Autodesk Inventor part; units mm, degrees
ref_plane "YZ Plane" through (0, 0, 0) normal (1, 0, 0) x (0, 1, 0)
ref_plane "XZ Plane" through (0, 0, 0) normal (0, 1, 0) x (-1, 0, 0)
ref_plane "XY Plane" through (0, 0, 0) normal (0, 0, 1) x (1, 0, 0)
sketch "Sketch1" plane through (0, 0, 0) normal (0, 0, 1) x (1, 0, 0)
  circle A0 centre (0, 0) radius 17.5
  circle A1 centre (0, 0) radius 67.5
  circle A2 centre (41.5, 0) radius 2
  circle A3 centre (29.3449, 29.3449) radius 2
  circle A4 centre (0, 41.5) radius 2
  circle A5 centre (-29.3449, 29.3449) radius 2
  circle A6 centre (-41.5, 0) radius 2
  circle A7 centre (-29.3449, -29.3449) radius 2
  circle A8 centre (0, -41.5) radius 2
  circle A9 centre (29.3449, -29.3449) radius 2
  dimension "d0" = 35
  dimension "d1" = 135
  dimension "d2" = 4
  dimension "d3" = 41.5
  dimension "d6" = 360
extrude "Extrusion1" add sketch "Sketch1" along normal blind 15
sketch "Sketch5" plane through (0, 0, 15) normal (0, 0, 1) x (1, 0, 0)
  circle A0 centre (0, 0) radius 67.5
  circle A1 centre (0, 0) radius 48.5
  dimension "d19" = 97
extrude "Extrusion4" add sketch "Sketch5" along normal blind 40
sketch "Sketch11" plane through (0, 0, 55) normal (0, 0, 1) x (1, 0, 0)
  line L0 (0, 77.9423) -> (67.5, 38.9711)
  line L1 (67.5, 38.9711) -> (67.5, -38.9711)
  line L2 (67.5, -38.9711) -> (0, -77.9423)
  line L3 (0, -77.9423) -> (-67.5, -38.9711)
  line L4 (-67.5, -38.9711) -> (-67.5, 38.9711)
  line L5 (-67.5, 38.9711) -> (0, 77.9423)
  circle A0 centre (0, 0) radius 67.5
extrude "Extrusion8" add sketch "Sketch11" against normal blind 55 contours L0 A0 L5 | L0 L1 A0 | A0 L4 L5 | L1 L2 A0 | A0 L3 L4 | L2 L3 A0
sketch "Sketch16" plane through (0, 0, 15) normal (0, 0, 1) x (1, 0, 0)
  circle A0 centre (-41.5, 0) radius 2
  circle A1 centre (0, 0) radius 34.5
  circle A2 centre (0, 0) radius 48.5
  line L0 (-48.5, 0) -> (-34.5, 0)
  circle A3 centre (0, 0) radius 48.5
extrude "Extrusion11" cut sketch "Sketch16" against normal blind 8
sketch "Sketch19" plane through (0, 0, 55) normal (0, 0, 1) x (1, 0, 0)
  circle A0 centre (0, 0) radius 48.5
  line L0 (0, -77.9423) -> (-67.5, -38.9711)
  line L1 (67.5, -38.9711) -> (0, -77.9423)
  line L2 (67.5, 38.9711) -> (67.5, -38.9711)
  line L3 (0, 77.9423) -> (67.5, 38.9711)
  line L4 (-67.5, 38.9711) -> (0, 77.9423)
  line L5 (-67.5, -38.9711) -> (-67.5, 38.9711)
  line L6 (0, 68.1273) -> (59, 34.0637)
  line L7 (59, 34.0637) -> (59, -34.0637)
  line L8 (59, -34.0637) -> (0, -68.1273)
  line L9 (0, -68.1273) -> (-59, -34.0637)
  line L10 (-59, -34.0637) -> (-59, 34.0637)
  line L11 (-59, 34.0637) -> (0, 68.1273)
  dimension "d58" = 118
extrude "Extrusion13" cut sketch "Sketch19" against normal through all contours L0 L5 L4 L3 L2 L1
sketch "Sketch20" plane through (0, 0, 0) normal (0, 0, -1) x (-1, 0, 0)
  line L0 (-59, -34.0637) -> (-59, -115)
  line L1 (-59, -115) -> (59, -115)
  line L2 (59, -34.0637) -> (59, 34.0637)
  line L3 (59, -115) -> (59, -34.0637)
  line L4 (-59, -34.0637) -> (0, -68.1273)
  line L5 (0, -68.1273) -> (59, -34.0637)
  line L6 (-59, -34.0637) -> (0, -68.1273)
  line L7 (0, -68.1273) -> (59, -34.0637)
  point P0 (0, 0)
  dimension "d61" = 115
extrude "Extrusion14" add sketch "Sketch20" against normal blind 55
sketch "Sketch22" plane through (0, 0, 55) normal (0, 0, 1) x (1, 0, 0)
  line L0 (59, -115) -> (59, 34.0637) construction
  line L1 (59, 34.0637) -> (0, 68.1273) construction
  line L2 (0, 68.1273) -> (-59, 34.0637) construction
  line L3 (-59, 34.0637) -> (-59, -115) construction
  line L4 (-59, -115) -> (59, -115) construction
  line L5 (52, 30.0222) -> (52, -108) construction
  line L6 (52, -108) -> (-52, -108) construction
  line L7 (-52, -108) -> (-52, 30.0222) construction
  line L8 (-52, 30.0222) -> (0, 60.0444) construction
  line L9 (0, 60.0444) -> (52, 30.0222) construction
  circle A0 centre (-52, -108) radius 2
  circle A1 centre (52, -108) radius 2
  circle A2 centre (0, 60.0444) radius 2
  circle A3 centre (-52, 30.0222) radius 2
  circle A4 centre (52, 30.0222) radius 2
  circle A5 centre (-26, -108) radius 2
  circle A6 centre (26, -108) radius 2
  circle A7 centre (0, -108) radius 2
  circle A8 centre (-52, -68.9889) radius 2
  circle A9 centre (-52, -38.9889) radius 2
  circle A10 centre (-52, 0) radius 2
  circle A11 centre (52, 0) radius 2
  circle A12 centre (52, -38.9889) radius 2
  circle A13 centre (52, -68.9889) radius 2
  circle A14 centre (-26, 45.0333) radius 2
  circle A15 centre (26, 45.0333) radius 2
  point P0 (0, 0)
  point P1 (0, 0)
  point P2 (0, 68.1273)
  point P3 (59, 34.0637)
  dimension "d64" = 7
  dimension "d65" = 4
  dimension "d66" = 4
  dimension "d67" = 4
  dimension "d68" = 4
  dimension "d69" = 4
  dimension "d70" = 4
  dimension "d71" = 4
  dimension "d72" = 4
  dimension "d73" = 4
  dimension "d74" = 4
  dimension "d75" = 4
  dimension "d76" = 4
  dimension "d77" = 4
  dimension "d78" = 4
  dimension "d79" = 4
  dimension "d80" = 4
  dimension "d81" = 30
extrude "Extrusion15" cut sketch "Sketch22" against normal through all contours A0 | A1 | A3 | A4 | A9 | A12 | A14 | A15
sketch "Sketch23" plane through (-59, -115, 0) normal (0, -1, 0) x (1, 0, 0)
  line L0 (12.812, 40) -> (35.906, 80)
  line L1 (35.906, 80) -> (82.094, 80)
  line L2 (82.094, 80) -> (105.188, 40)
  line L3 (105.188, 40) -> (82.094, 0)
  line L4 (82.094, 0) -> (35.906, 0)
  line L5 (35.906, 0) -> (12.812, 40)
  line L6 (118, 0) -> (0, 0)
  point P0 (59, 0)
  point P1 (59, 40)
  point P2 (59, 0)
  point P3 (59, 0)
  dimension "d87" = 80
extrude "Extrusion16" add sketch "Sketch23" along normal blind 13
sketch "Sketch24" plane through (-59, -128, 0) normal (0, -1, 0) x (1, 0, 0)
  line L0 (35.906, 80) -> (12.812, 40)
  line L1 (12.812, 40) -> (35.906, 0)
  line L2 (35.906, 0) -> (82.094, 0)
  line L3 (82.094, 0) -> (105.188, 40)
  line L4 (105.188, 40) -> (82.094, 80)
  line L5 (82.094, 80) -> (35.906, 80)
  line L6 (40.5248, 8) -> (22.0496, 40)
  line L7 (22.0496, 40) -> (40.5248, 72)
  line L8 (40.5248, 72) -> (77.4752, 72)
  line L9 (77.4752, 72) -> (95.9504, 40)
  line L10 (95.9504, 40) -> (77.4752, 8)
  line L11 (77.4752, 8) -> (40.5248, 8)
  point P0 (59, 0)
  dimension "d88" = 8
extrude "Extrusion17" cut sketch "Sketch24" against normal up to surface (13 mm away) from surface at 0
sketch "Sketch25" plane through (-59, -128, 0) normal (0, -1, 0) x (1, 0, 0)
  line L0 (95.9504, 40) -> (77.4752, 72)
  line L1 (77.4752, 72) -> (40.5248, 72)
  line L2 (40.5248, 72) -> (22.0496, 40)
  line L3 (22.0496, 40) -> (40.5248, 8)
  line L4 (40.5248, 8) -> (77.4752, 8)
  line L5 (77.4752, 8) -> (95.9504, 40)
  circle A0 centre (59, 40) radius 12
  point P0 (59, 0)
  point P1 (59, 72)
  dimension "d91" = 24
extrude "Extrusion18" cut sketch "Sketch25" against normal blind 40 contours A0
sketch "Sketch26" plane through (0, 0, 55) normal (0, 0, 1) x (1, 0, 0)
  line L0 (12, -88) -> (-12, -88)
  line L1 (12, -128) -> (-12, -128)
  line L2 (12, -88) -> (-12, -88)
  line L3 (-12, -88) -> (12, -88)
  line L4 (12, -88) -> (12, -101)
  line L5 (12, -101) -> (-12, -101)
  line L6 (-12, -101) -> (-12, -88)
  point P0 (0, 0)
  dimension "d94" = 13
extrude "Extrusion19" cut sketch "Sketch26" against normal blind 15
sketch "Sketch27" plane through (-36.9504, -128, 40) normal (-0.866, 0, 0.5) x (0.5, 0, 0.866)
  line L0 (17.3205, 13) -> (36.9504, 13)
  line L1 (17.3205, 13) -> (0, 13)
  line L2 (0, 0) -> (0, 13)
  line L3 (36.9504, 0) -> (0, 0)
  line L4 (36.9504, 0) -> (36.9504, 13)
  circle A0 centre (11.4041, 4) radius 2
  circle A1 centre (25.5463, 9) radius 2
  line L5 (11.4041, 4) -> (25.5463, 9) construction
  line L6 (0, 13) -> (36.9504, 13)
  point P0 (-16.1658, 128)
  point P1 (18.4752, 6.5)
  point P2 (18.4752, 13)
  point P3 (0, 6.5)
  dimension "d97" = 4
  dimension "d98" = 4
  dimension "d99" = 15
  dimension "d112" = 5
extrude "Extrusion20" cut sketch "Sketch27" against normal blind 20 contours A0 | A1
pattern_circular "Circular Pattern1" count 6 over 360 about axis through (0, -128, 40) along (0, 1, 0) of "Extrusion20"
sketch "Sketch28" plane through (0, 0, 55) normal (0, 0, 1) x (1, 0, 0)
  circle A0 centre (0, 53.1273) radius 2
  circle A1 centre (-34, -90) radius 2
  line L0 (-59, 34.0637) -> (-59, -115)
  line L1 (-59, -115) -> (-28.2902, -115)
  point P0 (0, 0)
  point P1 (0, 68.1273)
  dimension "d105" = 4
  dimension "d106" = 15
  dimension "d107" = 4
  dimension "d108" = 25
  dimension "d109" = 25
extrude "Extrusion21" cut sketch "Sketch28" against normal through all
sketch "Sketch30" plane through (0, 0, 55) normal (0, 0, 1) x (1, 0, 0)
  circle A0 centre (0, 0) radius 48.5 construction
  line L0 (12, -88) -> (12, -101) construction
  line L1 (12, -88) -> (-12, -88) construction
  line L2 (-12, -88) -> (-12, -101) construction
  line L3 (-12, -101) -> (12, -101) construction
  line L4 (12, -128) -> (-12, -128) construction
  circle A1 centre (-34, -90) radius 2 construction
  line L5 (-17, -83) -> (17, -83) construction
  line L6 (17, -83) -> (17, -106) construction
  line L7 (17, -106) -> (-17, -106) construction
  line L8 (-17, -106) -> (-17, -83) construction
  circle A2 centre (-34, -90) radius 7 construction
  circle A3 centre (0, 0) radius 53.5 construction
  circle A4 centre (0, 53.1273) radius 2 construction
  circle A5 centre (-34, -90) radius 2 construction
  line L9 (-12, -101) -> (-12, -88) construction
  line L10 (-12, -88) -> (12, -88) construction
  line L11 (12, -88) -> (12, -101) construction
  line L12 (12, -101) -> (-12, -101) construction
  circle A6 centre (26, 45.0333) radius 2 construction
  circle A7 centre (-52, 30.0222) radius 2 construction
  circle A8 centre (-52, -108) radius 2 construction
  circle A9 centre (52, -38.9889) radius 2 construction
  circle A10 centre (52, -108) radius 2 construction
  circle A11 centre (-52, -38.9889) radius 2 construction
  circle A12 centre (-26, 45.0333) radius 2 construction
  circle A13 centre (52, 30.0222) radius 2 construction
  line L13 (0, 68.1273) -> (-59, 34.0637) construction
  line L14 (-59, 34.0637) -> (-59, -115) construction
  line L15 (-59, -115) -> (-28.2902, -115) construction
  line L16 (-28.2902, -115) -> (28.2902, -115) construction
  line L17 (28.2902, -115) -> (59, -115) construction
  line L18 (59, -115) -> (59, 34.0637) construction
  line L19 (59, 34.0637) -> (0, 68.1273) construction
  circle A14 centre (0, 0) radius 48.5 construction
  line L20 (-46, -102) -> (-46, 26.5581) construction
  line L21 (-46, 26.5581) -> (0, 53.1162) construction
  line L22 (0, 53.1162) -> (46, 26.5581) construction
  line L23 (46, 26.5581) -> (46, -102) construction
  line L24 (46, -102) -> (28.2902, -102) construction
  line L25 (28.2902, -102) -> (-28.2902, -102) construction
  line L26 (-28.2902, -102) -> (-46, -102) construction
  line L27 (-23, -50.9295) -> (-8, -59.5897)
  line L28 (-8, -59.5897) -> (-8, -76.9103)
  line L29 (-8, -76.9103) -> (-23, -85.5705)
  line L30 (-23, -85.5705) -> (-38, -76.9103)
  line L31 (-38, -76.9103) -> (-38, -59.5897)
  line L32 (-38, -59.5897) -> (-23, -50.9295)
  line L33 (23, -50.9295) -> (38, -59.5897)
  line L34 (38, -59.5897) -> (38, -76.9103)
  line L35 (38, -76.9103) -> (23, -85.5705)
  line L36 (23, -85.5705) -> (8, -76.9103)
  line L37 (8, -76.9103) -> (8, -59.5897)
  line L38 (8, -59.5897) -> (23, -50.9295)
  line L39 (0, -83) -> (-46, -83) construction
  line L40 (0, -83) -> (46, -83) construction
  line L41 (0, -53.5) -> (0, -83) construction
  point P0 (-23, -68.25)
  point P1 (23, -68.25)
  point P2 (-23, -83)
  point P3 (23, -83)
  point P4 (0, -68.25)
  dimension "d121" = 5
  dimension "d122" = 5
  dimension "d123" = 5
  dimension "d124" = 13
  dimension "d125" = 30
extrude "Extrusion23" [suppressed]
sketch "Sketch31" plane through (0, 0, 5) normal (0, 0, 1) x (1, 0, 0)
  line L0 (-52.3536, -52.747) -> (-52.3536, -97.747)
  line L1 (-52.3536, -97.747) -> (-41.747, -108.3536)
  line L2 (-41.747, -108.3536) -> (-26.747, -108.3536)
  circle A0 centre (-52, -108) radius 2
  line L3 (-52, -108) -> (-47.0503, -103.0503)
  line L4 (-26.747, -98.3536) -> (-37.6048, -98.3536)
  line L5 (-37.6048, -98.3536) -> (-42.3536, -93.6048)
  line L6 (-42.3536, -93.6048) -> (-42.3536, -52.747)
  line L7 (-52.3536, -52.747) -> (-42.3536, -52.747)
  line L8 (-26.747, -98.3536) -> (-26.747, -108.3536)
  point P0 (0, 0)
  dimension "d128" = 45
  dimension "d129" = 15
  dimension "d130" = 15
  dimension "d131" = 135
  dimension "d132" = 7
  dimension "d133" = 10
extrude "Extrusion24" [suppressed]
mirror "Mirror1" [suppressed]
sketch "Sketch32" plane through (0, 0, 0) normal (0, 0, -1) x (-1, 0, 0)
  circle A0 centre (0, 0) radius 33
  dimension "d139" = 66
extrude "Extrusion25" cut sketch "Sketch32" against normal blind 2
properties part number "AC01" material "ABS Plastic"
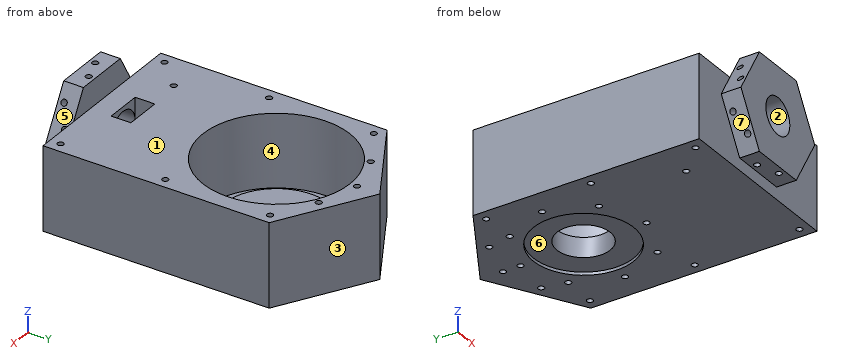
Part model, mm, in its own coordinate system. Face numbers are marked on the shaded views. A direction names the side the tool comes from. Round coordinates to 2 decimals unless told otherwise and drop trailing zeros. Write each loop counter-clockwise with the first axis right and the second up, starting at its lowest first coordinate (ties: lowest second). Pieces come first, ordered by that corner, then holes. Notation, with made-up numbers: (85.5, 58) -> (138.5, 58) arc R17 cw to (138.5, 73) -> close; hole circle Ø8 at (-28, 12.25). An arc over 180 degrees is marked (long way). Return JSON: item names as keys, results as strings. Group by question number.
Q1. Saw through at B-B on z = 10. State how many separate pieces and enclosed holes the cut face has, plus the area to 3 significant figures.
Q2. Pin check, flat tips, straight feed: pin 1 (14.5 mm diameter, centred on x = 0, z = 40, fed in from -Y); pin 2 (3 mm diameter, centred on x = -52, y = -108, fed in from +Z); pin 3 (2 mm diameter, centred on x = 26.5, z = 39, fed in from +Y); pin 4 (12 mm diameter, centred on x = 15, y = 35.5, fed in from +Z). Stop position of each tip, or through.
Q3. Saw through at C-C on y = 0. Write the cut outline in (x, z), plus the area to 3 significant figures.
Q4. Mould opens along Z. For the marked faces 1, 2 and 3 say: pulls with the +Z half, pulls with the -Z half, needs draft (parallel to the pull), parting line crosses it, or undercut.
Q5. Saw through at D-D on x = -41.5. Write the cut outline in (y, z).
Q6. Which spindle directions (+Z, -Z, +X, -X, +Y, -Y) get a long thin tool onto all of the face, cutting with end or side? Do the marked faces 4, 5, 6 and 7. Say none if no direction does.
Q7. Probe L1, parallel to Y at x = 0, z = 1.5; L2, parallel to Y at x = -52, z = 14; L3, parallel to Y at x = -26, z = 38. List the from-to ranges inside material, lowest first. Write a range as [from, to].
Q8. Saw through at A-A on y = -108. Write the cut outline in (x, z), plus the area to 3 significant figures.
Answer:
{
 "1": {"separate pieces": "2", "enclosed holes": "14", "area": "15,300 mm2"},
 "2": {"pin 1": "y = -88", "pin 2": "through", "pin 3": "y = 53.4", "pin 4": "z = 15"},
 "3": {"outline": "(-59, 0) -> (-43.5, 0) -> (-43.5, 7) -> (-48.5, 7) -> (-48.5, 55) -> (-59, 55) -> close; (-39.5, 0) -> (-33, 0) -> (-33, 2) -> (-17.5, 2) -> (-17.5, 15) -> (-34.5, 15) -> (-34.5, 7) -> (-39.5, 7) -> close; (17.5, 2) -> (33, 2) -> (33, 0) -> (39.5, 0) -> (39.5, 7) -> (34.5, 7) -> (34.5, 15) -> (17.5, 15) -> close; (43.5, 0) -> (59, 0) -> (59, 55) -> (48.5, 55) -> (48.5, 7) -> (43.5, 7) -> close", "area": "1,740 mm2"},
 "4": {"face 1": "pulls with the +Z half", "face 2": "undercut", "face 3": "needs draft"},
 "5": {"outline": "(-115, 0) -> (-2, 0) -> (-2, 7) -> (-25.1, 7) -> (-25.1, 55) -> (-115, 55) -> close; (2, 0) -> (44.17, 0) -> (44.17, 55) -> (25.1, 55) -> (25.1, 7) -> (2, 7) -> close"},
 "6": {"face 4": "+Z", "face 5": "+Z, +X, -Y", "face 6": "-Z", "face 7": "-Z, -X, -Y"},
 "7": {"L1": "[-115, -43.5], [-39.5, -33], [33, 39.5], [43.5, 51.13], [55.13, 68.13]", "L2": "[-115, -110], [-106, -40.99], [-36.99, 28.02], [32.02, 38.11]", "L3": "[-128, -40.94], [40.94, 43.03], [47.03, 53.12]"},
 "8": {"outline": "(-59, 0) -> (-54, 0) -> (-54, 55) -> (-59, 55) -> close; (-50, 0) -> (50, 0) -> (50, 55) -> (-50, 55) -> close; (54, 0) -> (59, 0) -> (59, 55) -> (54, 55) -> close; hole circle Ø24 at (0, 40)", "area": "5,600 mm2"}
}
